```python
from build123d import *

# Parameters (mm, degrees)
EXTRUDE_1_DEPTH          = 2000
CUT_EXTRUDE_1_DEPTH      = 2001.112496836
CUT_EXTRUDE_1_DEPTH_BACK = 2001.112496836
SKETCH_2_R               = 5


with BuildPart() as part:
    # Эскиз1 → Бобышка-Вытянуть1 (new body)
    with BuildSketch(Plane(origin=(0, 0, 0), x_dir=(1, 0, 0), z_dir=(0, 1, 0))):
        with BuildLine():
            Line((-12, 15), (12, 15))
            ThreePointArc((12, 15), (14.121320344, 14.121320344), (15, 12))
            Line((15, 12), (15, -12))
            ThreePointArc((15, -12), (14.121320344, -14.121320344), (12, -15))
            Line((12, -15), (-12, -15))
            ThreePointArc((-12, -15), (-14.121320344, -14.121320344), (-15, -12))
            Line((-15, -12), (-15, 12))
            ThreePointArc((-15, 12), (-14.121320344, 14.121320344), (-12, 15))
        make_face()
        with BuildLine():
            Line((-11, 13), (11, 13))
            ThreePointArc((11, 13), (12.414213562, 12.414213562), (13, 11))
            Line((13, 11), (13, -11))
            ThreePointArc((13, -11), (12.414213562, -12.414213562), (11, -13))
            Line((11, -13), (-11, -13))
            ThreePointArc((-11, -13), (-12.414213562, -12.414213562), (-13, -11))
            Line((-13, -11), (-13, 11))
            ThreePointArc((-13, 11), (-12.414213562, 12.414213562), (-11, 13))
        make_face(mode=Mode.SUBTRACT)
    extrude(amount=EXTRUDE_1_DEPTH)

    # Эскиз2 → Вырез-Вытянуть1 (cut, two sides: drawn at the far end of the back side and taken through both)
    with BuildSketch(Plane(origin=(0, 0, 0), x_dir=(0, 0, -1), z_dir=(1, 0, 0)).offset(-CUT_EXTRUDE_1_DEPTH_BACK)):
        with Locations((0, 100)):
            Circle(SKETCH_2_R)
        with Locations((0, 200)):
            Circle(SKETCH_2_R)
        with Locations((0, 300)):
            Circle(SKETCH_2_R)
        with Locations((0, 400)):
            Circle(SKETCH_2_R)
        with Locations((0, 500)):
            Circle(SKETCH_2_R)
        with Locations((0, 600)):
            Circle(SKETCH_2_R)
        with Locations((0, 700)):
            Circle(SKETCH_2_R)
        with Locations((0, 800)):
            Circle(SKETCH_2_R)
        with Locations((0, 900)):
            Circle(SKETCH_2_R)
        with Locations((0, 1000)):
            Circle(SKETCH_2_R)
        with Locations((0, 1100)):
            Circle(SKETCH_2_R)
        with Locations((0, 1200)):
            Circle(SKETCH_2_R)
        with Locations((0, 1300)):
            Circle(SKETCH_2_R)
        with Locations((0, 1400)):
            Circle(SKETCH_2_R)
        with Locations((0, 1500)):
            Circle(SKETCH_2_R)
        with Locations((0, 1600)):
            Circle(SKETCH_2_R)
        with Locations((0, 1700)):
            Circle(SKETCH_2_R)
        with Locations((0, 1800)):
            Circle(SKETCH_2_R)
    extrude(amount=CUT_EXTRUDE_1_DEPTH + CUT_EXTRUDE_1_DEPTH_BACK, mode=Mode.SUBTRACT)


solid = part.part
```
Build history of the part. All positions in model axes, mm. Round coordinates to 2 decimals unless told otherwise and drop trailing zeros. Write each loop counter-clockwise with the first axis right and the second up, starting at its lowest first coordinate (ties: lowest second). Pieces come first, ordered by that corner, then holes. Notation, with made-up numbers: (-15, 67.25) - (39, 67.25) arc R14 cw to (39, 83.25) - close; hole circle Ø2 at (56.5, -34). An arc over 180 degrees is marked (long way). Write each question's results on one line, items separated by ' | '. Start each with the question number.
Item 1: Saw through at C-C (z = -0.5). State how many separate pieces and enclosed holes the cut face has, and give its area (3 significant figures).
Item 2: Saw through at A-A (x = 2.25). Write the cut outline in (y, z), and give its area (3 significant figures).
Item 3: Wall check: L1, parallel to X at y = 493, z = -5.5; L2, parallel to X at y = 1105, z = -12.5. Give the ranges that are in metal, low to high. Write a range as [from, to].
Item 4: Saw through at B-B (y = 1461.5). Write the cut outline in (x, z), and give its area (3 significant figures).
Results are:
1) separate pieces: 38 | enclosed holes: 0 | area: 7,280 mm²
2) outline: (0, -15) - (2000, -15) - (2000, -13) - (0, -13) - close; (0, 13) - (2000, 13) - (2000, 15) - (0, 15) - close | area: 8,000 mm²
3) L1: x = [-15, -13], [13, 15] | L2: x = [-14.96, -12.32], [12.32, 14.96]
4) outline: (-15, -12) arc R3 ccw to (-12, -15) - (12, -15) arc R3 ccw to (15, -12) - (15, 12) arc R3 ccw to (12, 15) - (-12, 15) arc R3 ccw to (-15, 12) - close; hole (-13, -11) arc R2 ccw to (-11, -13) - (11, -13) arc R2 ccw to (13, -11) - (13, 11) arc R2 ccw to (11, 13) - (-11, 13) arc R2 ccw to (-13, 11) - close | area: 220 mm²
